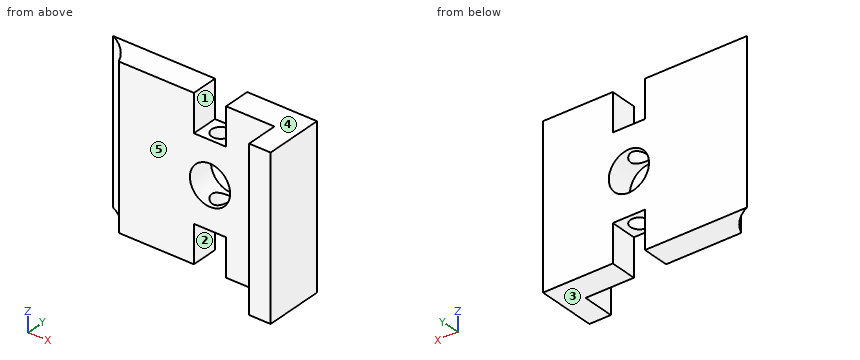
from build123d import *

# Parameters (mm, degrees)
BOSS_EXTRUDE1_DEPTH = 14.835
CUT_EXTRUDE1_REACH  = 37.321
SKETCH4_R           = 1.65
SKETCH4_3_W         = 6
SKETCH4_3_H         = 5
SKETCH4_3_R         = 1.65
CUT_EXTRUDE3_DEPTH  = 7
CUT_EXTRUDE2_REACH  = 26.619
SKETCH5_R           = 3.75
SKETCH6_W           = 4
SKETCH6_H           = 6
BOSS_EXTRUDE2_DEPTH = 29.67


with BuildPart() as part:
    # Sketch3 → Boss-Extrude1 (new, symmetric)
    with BuildSketch(Plane.XY):
        with BuildLine():
            Line((-14, -2.5), (19, -2.5))
            Line((19, -2.5), (19, 2.5))
            Line((19, 2.5), (-19, 2.5))
            ThreePointArc((-19, 2.5), (-16.043310466, 0.456689534), (-14, -2.5))
        make_face()
    extrude(amount=BOSS_EXTRUDE1_DEPTH, both=True)

    # Sketch4 → Cut-Extrude1 (cut, up to next)
    with BuildSketch(Plane.XY.offset(14.835), mode=Mode.PRIVATE) as cut_extrude1_sk1:
        with Locations((3, 0)):
            Circle(SKETCH4_R)
    cut_extrude1_tool1 = extrude(cut_extrude1_sk1.sketch, amount=-CUT_EXTRUDE1_REACH, mode=Mode.PRIVATE) & part.part
    add(cut_extrude1_tool1.solids().sort_by_distance((3, 0, 14.835))[0], mode=Mode.SUBTRACT)

    # Sketch4<3> → Cut-Extrude3 (cut)
    with BuildSketch(Plane.XY.offset(14.835)):
        with Locations((3, 0)):
            Rectangle(SKETCH4_3_W, SKETCH4_3_H)
        with Locations((3, 0)):
            Circle(SKETCH4_3_R, mode=Mode.SUBTRACT)
    cut_extrude3 = extrude(amount=-CUT_EXTRUDE3_DEPTH, mode=Mode.SUBTRACT)

    # Mirror1: Cut-Extrude3 across plane
    add(cut_extrude3.mirror(Plane.XY), mode=Mode.SUBTRACT)

    # Sketch5 → Cut-Extrude2 (cut, up to next)
    with BuildSketch(Plane(origin=(0, 2.5, 0), x_dir=(1, 0, 0), z_dir=(0, 1, 0)), mode=Mode.PRIVATE) as cut_extrude2_sk1:
        with Locations(Location((3, 0, 0), (0, 0, 270))):
            Circle(SKETCH5_R)
    cut_extrude2_tool1 = extrude(cut_extrude2_sk1.sketch, amount=-CUT_EXTRUDE2_REACH, mode=Mode.PRIVATE) & part.part
    add(cut_extrude2_tool1.solids().sort_by_distance((3, 2.5, 0))[0], mode=Mode.SUBTRACT)

    # Sketch6 → Boss-Extrude2 (add)
    with BuildSketch(Plane.XY.offset(14.835)):
        with Locations((17, -5.5)):
            Rectangle(SKETCH6_W, SKETCH6_H)
    extrude(amount=-BOSS_EXTRUDE2_DEPTH)


solid = part.part
Check sheet for the modelled part. Datum: model origin and axes. Units: mm. Face numbers are marked on the shaded views. A direction names the side the tool comes from. Round coordinates to 2 decimals unless told otherwise and drop trailing zeros. Order: outer loops, then holes, each group sorted by start corner. A loop starts at its lowest first (then second) coordinate and runs counter-clockwise, first axis right, second up.
(1) Go/stop test with flat-tipped pins: P1, Ø5.5, axis at y = 0.5, z = 11.5, coming from the -X side; P2, Ø3, axis at y = -2, z = -1.5, coming from the -X side; P3, Ø4, axis at x = 3.5, y = 0.5, coming from the -Z side (3 decimals); P4, Ø1.8, axis at y = -4, z = 3.5, coming from the -X side. Record where each tip stops, or that it passes through.
(2) Cross-section at B-B, the plane x = 3. Enter the section's corners in (y, z) (3 decimals), and give its area (3 significant figures).
(3) Access from +Z, -Z, +X, -X, +Y, -Y to the whole of each face (thin tool, end or side, straight path). Record for the marked faces 1, 2, 3, 4 and 5.
(4) Scan lines: probe 1 along X at (y, z) = (-1, 0); probe 2 along Y at (x, z) = (3, 5.8); probe 3 along X at (y, z) = (1.1, 0). Record each from-to range of solid material in increasing order.
(5) Cross-section at A-A, the plane z = 0. Enter the section's corners in (x, y).
(6) Cross-section at D-D, the plane z = 12.75. Enter the section's corners in (x, y), and give its area (3 significant figures).
Check sheet entries:
1. P1: stops at x = -19
1. P2: stops at x = -15.2
1. P3: stops at z = -7.835
1. P4: stops at x = 15
2. outline: (-2.5, -7.835) - (-1.65, -7.835) - (-1.65, -3.75) - (-2.5, -3.75) - close; (-2.5, 3.75) - (-1.65, 3.75) - (-1.65, 7.835) - (-2.5, 7.835) - close; (1.65, -7.835) - (2.5, -7.835) - (2.5, -3.75) - (1.65, -3.75) - close; (1.65, 3.75) - (2.5, 3.75) - (2.5, 7.835) - (1.65, 7.835) - close
2. area: 13.9 mm2
3. face 1: +Z, +Y, -Y
3. face 2: -Z, +Y, -Y
3. face 3: -Z, +X, -X, +Y, -Y
3. face 4: +Z, +X, -X, +Y, -Y
3. face 5: +Z, -Z, -X, -Y
4. probe 1: x = -14.84 to -0.75, 6.75 to 19
4. probe 2: y = -2.5 to -1.65, 1.65 to 2.5
4. probe 3: x = -16.75 to -0.75, 6.75 to 19
5. outline: (-19, 2.5) arc R10 cw to (-14, -2.5) - (-0.75, -2.5) - (-0.75, 2.5) - close; (6.75, -2.5) - (15, -2.5) - (15, -8.5) - (19, -8.5) - (19, 2.5) - (6.75, 2.5) - close
6. outline: (-19, 2.5) arc R10 cw to (-14, -2.5) - (0, -2.5) - (0, 2.5) - close; (6, -2.5) - (15, -2.5) - (15, -8.5) - (19, -8.5) - (19, 2.5) - (6, 2.5) - close
6. area: 168 mm2
